Autodesk Inventor part; units mm, degrees
ref_plane "YZ Plane" through (0, 0, 0) normal (1, 0, 0) x (0, 1, 0)
ref_plane "XZ Plane" through (0, 0, 0) normal (0, 1, 0) x (-1, 0, 0)
ref_plane "XY Plane" through (0, 0, 0) normal (0, 0, 1) x (1, 0, 0)
sketch "Boceto1" plane through (0, 0, 0) normal (0, 0, 1) x (1, 0, 0)
  arc A0 (8.1351, 6.7837) -> (8.1351, -10.1182) centre (11.2305, -1.6673) ccw
  line L0 (8.1351, 6.7837) -> (8.1351, -10.1182)
  point P0 (0, 0)
  dimension "d2" = 18
extrude "Extrusión1" add sketch "Boceto1" along normal blind 8
fillet "Empalme3" radius 0.5 1 edges at (8.1351, 6.7837, 4)
fillet "Empalme4" radius 0.5 1 edges at (8.1351, -10.1182, 4)
sketch "Boceto4" plane through (8.1351, 6.0349, 8) normal (1, 0, 0) x (0, 0, -1)
  line L0 (8, 0.4531) -> (0, 0.4531)
  line L1 (4, 0.4531) -> (4, -7.7019)
  line L2 (0, -15.8574) -> (8, -15.8574)
  circle A0 centre (4, -7.7019) radius 4
  point P0 (8, -6.0349)
  dimension "d29" = 8.155
  dimension "d30" = 8
extrude "Extrusión4" add sketch "Boceto4" along normal blind 3
sketch "Boceto5" plane through (11.1351, -1.6671, 4) normal (1, 0, 0) x (0, 0, -1)
  circle A0 centre (0, 0) radius 3.375
  point P0 (4, 1.6671)
  dimension "d33" = 6.75
extrude "Extrusión5" add sketch "Boceto5" along normal blind 19
chamfer "Chaflán2" distance 1 angle 45 1 edges at (30.1351, -1.6671, 7.375)
sketch "Boceto6" plane through (0, 0, 8) normal (0, 0, 1) x (1, 0, 0)
  point P0 (0, 0)
properties part number "Tornillo" material "Acero inoxidable"
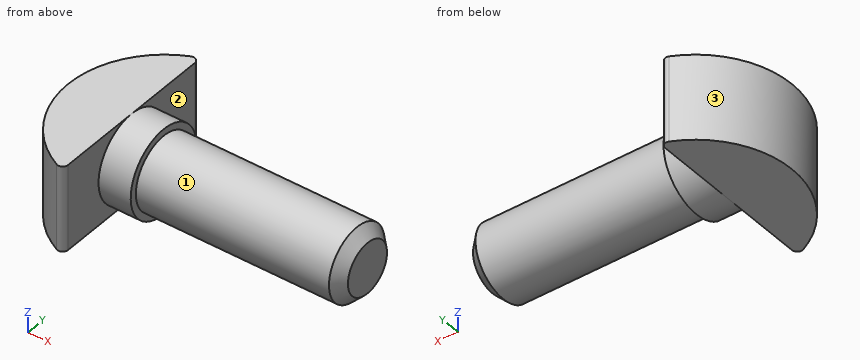
The listing builds one solid part. Answer for the finished solid, in the listing's coordinates (mm). Face numbers are marked on the shaded views. A direction names the side the tool comes from. Give positions to 0.01 mm unless a question says otherwise; leave off trailing zeros. Loops run counter-clockwise (first coordinate to the right, second up) from the corner with the lowest first, then second, coordinate; pieces in that order, holes last. Notation, with made-up numbers: (-11.5, 0.25) - (38.5, 0.25) arc R27 ccw to (38.5, 38.25) - close; hole circle Ø4 at (11.25, -27.75). An arc over 180 degrees is marked (long way). Return JSON: item names as keys, results as strings. Group by question number.
1. Which of the six approach directions +Z, -Z, +X, -X, +Y, -Y give full straight-line access (tool end or side, diameter ignored) to the marked faces 1, 2 and 3?
2. Find section D-D (x = 28.25). Write down the section's boundary in (y, z) (3 decimals), then the cut area to 3 significant figures.
3. Find section C-C (y = -6.25). Write down the section's boundary in (x, z), then the cut area to 3 significant figures.
4. Straight lines are drawn through the part: line 1 (Y direction, x = 25.75, z = 4); line 2 (Y direction, x = 25.75, z = 2); line 3 (X direction, y = -7, z = 2.75). For each, find the intervals that lie inside material, in ascending order. Write a range as [from, to].
5. Find section B-B (x = 5). Write down the section's boundary in (y, z), then the cut area to 3 significant figures.
6. Given pin 1 Ø4 at (y, z) = (-4, 3.5) entering from -X; pin 2 Ø4 at (x, y) = (26, -3.5) entering from +Z (3 decimals); pin 3 Ø2 at (x, z) = (10, 7) entering from +Y, each flat-ended and moving along its own axis, determine where each tip first touches the part or whether it passes through.
7. Find section A-A (z = 4). Write down the section's boundary in (x, y).
Verdict:
{
 "1": {"face 1": "+X", "face 2": "+X, +Y", "face 3": "+Z, -Z, -X"},
 "2": {"outline": "circle Ø6.75 at (-1.667, 4)", "area": "35.8 mm^2"},
 "3": {"outline": "(3.48, 0) - (8.14, 0) - (8.14, 8) - (3.48, 8) - close", "area": "37.2 mm^2"},
 "4": {"line 1": "y = [-5.04, 1.71]", "line 2": "y = [-4.39, 1.05]", "line 3": "x = [3.98, 8.14]"},
 "5": {"outline": "(-8.16, 0) - (4.83, 0) - (4.83, 8) - (-8.16, 8) - close", "area": "104 mm^2"},
 "6": {"pin 1": "stops at x = 2.24", "pin 2": "stops at z = 7.375", "pin 3": "stops at y = 1.8"},
 "7": {"outline": "(7.42, -9.82) arc R0.5 ccw to (8.14, -9.37) - (8.14, -5.67) - (11.14, -5.67) - (11.14, -5.04) - (29.14, -5.04) - (30.14, -4.04) - (30.14, 0.71) - (29.14, 1.71) - (11.14, 1.71) - (11.14, 2.33) - (8.14, 2.33) - (8.14, 6.03) arc R0.5 ccw to (7.42, 6.49) arc R9 ccw to start"}
}
